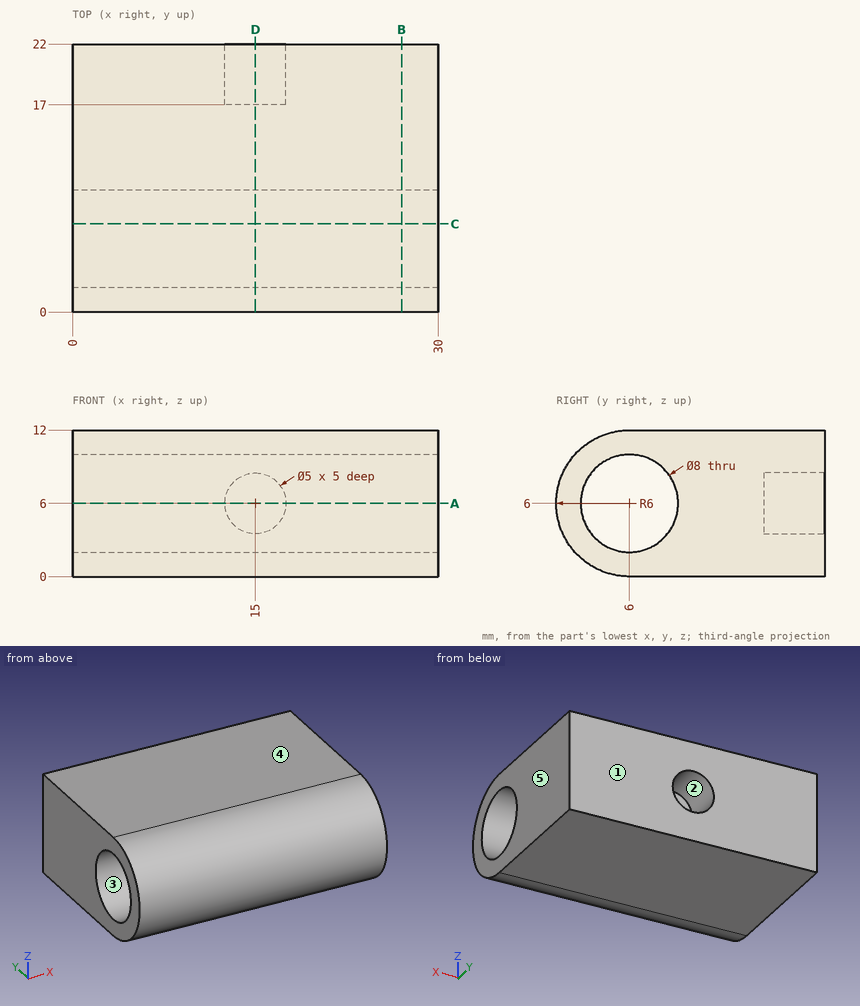
Check sheet for the drawn part. Datum: minimum x, y, z corner. Units: mm. A direction names the side the tool comes from. Coordinates: 2 decimals unless noted, no trailing zeros. Write each loop counter-clockwise with the first axis right and the second up, starting at its lowest first coordinate (ties: lowest second). Pieces come first, ordered by that corner, then holes. Notation, with made-up numbers: (64.5, 3.5) - (95.5, 3.5) arc R9 ccw to (95.5, 15.5) - close; hole circle Ø4 at (42.25, 86.25). An arc over 180 degrees is marked (long way). Answer as a JSON object with one key per item and string values.
(1) Cross-section at A-A on z = 6. Record the cut outline in (x, y).
Report:
{"outline": "(0, 0) - (30, 0) - (30, 2) - (0, 2) - close; (0, 10) - (30, 10) - (30, 22) - (17.5, 22) - (17.5, 17) - (12.5, 17) - (12.5, 22) - (0, 22) - close"}
(2) Thickness scan on line 1 along X through (y, z) = (18.9, 6); line 2 along Y through (x, z) = (13.25, 6); line 3 along Y through (x, z) = (1.5, 9.5). Record the ranges inside material, lowest first.
Report:
{"line 1": "0 to 12.5, 17.5 to 30", "line 2": "0 to 2, 10 to 17", "line 3": "1.13 to 4.06, 7.94 to 22"}
(3) Gauge pin test, flat ends, axial feed: pin 1 Ø7 at (y, z) = (6, 6) entering from -X; pin 2 Ø4.5 at (x, z) = (15, 6) entering from +Y. Record the tip position at first contact, or that the pin passes through.
Report:
{"pin 1": "through", "pin 2": "y = 17"}
(4) Tool access check on the marked faces 1 and 2. Record the directions out of +Z, -Z, +X, -X, +Y, -Y that give a thin tool (end or side, any length) a straight path to the whole face; none if there is none.
Report:
{"face 1": "+Z, -Z, +X, -X, +Y", "face 2": "+Y"}
(5) Cross-section at D-D on x = 15. Record the cut outline in (y, z).
Report:
{"outline": "(6, 0) - (22, 0) - (22, 3.5) - (17, 3.5) - (17, 8.5) - (22, 8.5) - (22, 12) - (6, 12) arc R6 ccw to start; hole circle Ø8 at (6, 6)"}
(6) Mould release check, pull along Z, two halves, no side actions. Record for the marked faces 3, 4 and 5: pulls with the +Z half, pulls with the -Z half, needs draft (parallel to the pull), parting line crosses it, or undercut.
Report:
{"face 3": "undercut", "face 4": "pulls with the +Z half", "face 5": "needs draft"}
(7) Cross-section at B-B on x = 27. Record the cut outline in (y, z), plus the area to 3 significant figures.
Report:
{"outline": "(6, 0) - (22, 0) - (22, 12) - (6, 12) arc R6 ccw to start; hole circle Ø8 at (6, 6)", "area": "198 mm^2"}
(8) Cross-section at C-C on y = 7.25. Record the cut outline in (x, z).
Report:
{"outline": "(0, 0) - (30, 0) - (30, 2.2) - (0, 2.2) - close; (0, 9.8) - (30, 9.8) - (30, 12) - (0, 12) - close"}
